from build123d import *

# Parameters (mm, degrees)
F0_W     = 200.66
F0_H     = 200.66
F1_DEPTH = 3.175


# Not quite as in the source:
# - a length typed as a fraction of an inch, garbled in the dataset ("3 / 203.2 mm" for 3/8 in), is restored


with BuildPart() as f1:
    # F0 (on Top) → F1 (new body)
    with BuildSketch(Plane.XY):
        Rectangle(F0_W, F0_H)
        with BuildLine():
            Line((-6.4755703305, -37.973), (-6.4755703305, -38.227))
            ThreePointArc((-6.4755703305, -38.227), (-14.2002143688, -48.9498629888), (-26.715108043, -44.704))
            Line((-26.715108043, -44.704), (-30.0367761716, -44.704))
            Line((-30.0367761716, -44.704), (-44.4783061624, -44.704))
            ThreePointArc((-44.4783061624, -44.704), (-49.0582367841, -42.8069306217), (-50.9553061624, -38.227))
            Line((-50.9553061624, -38.227), (-50.9553061624, -37.973))
            ThreePointArc((-50.9553061624, -37.973), (-49.0582367841, -33.3930693783), (-44.4783061624, -31.496))
            Line((-44.4783061624, -31.496), (-30.0367761716, -31.496))
            Line((-30.0367761716, -31.496), (-26.715108043, -31.496))
            ThreePointArc((-26.715108043, -31.496), (-14.2002143688, -27.2501370112), (-6.4755703305, -37.973))
        make_face(mode=Mode.SUBTRACT)
        with BuildLine():
            Line((82.4244296695, -37.973), (82.4244296695, -38.227))
            ThreePointArc((82.4244296695, -38.227), (74.6997856312, -48.9498629888), (62.184891957, -44.704))
            Line((62.184891957, -44.704), (58.8632238284, -44.704))
            Line((58.8632238284, -44.704), (44.4216938376, -44.704))
            ThreePointArc((44.4216938376, -44.704), (39.8417632159, -42.8069306217), (37.9446938376, -38.227))
            Line((37.9446938376, -38.227), (37.9446938376, -37.973))
            ThreePointArc((37.9446938376, -37.973), (39.8417632159, -33.3930693783), (44.4216938376, -31.496))
            Line((44.4216938376, -31.496), (58.8632238284, -31.496))
            Line((58.8632238284, -31.496), (62.184891957, -31.496))
            ThreePointArc((62.184891957, -31.496), (74.6997856312, -27.2501370112), (82.4244296695, -37.973))
        make_face(mode=Mode.SUBTRACT)
        with BuildLine():
            ThreePointArc((-50.9553061624, 38.227), (-49.0582367841, 42.8069306217), (-44.4783061624, 44.704))
            Line((-44.4783061624, 44.704), (-30.0367761716, 44.704))
            Line((-30.0367761716, 44.704), (-26.715108043, 44.704))
            ThreePointArc((-26.715108043, 44.704), (-14.2002143688, 48.9498629888), (-6.4755703305, 38.227))
            Line((-6.4755703305, 38.227), (-6.4755703305, 37.973))
            ThreePointArc((-6.4755703305, 37.973), (-14.2002143688, 27.2501370112), (-26.715108043, 31.496))
            Line((-26.715108043, 31.496), (-30.0367761716, 31.496))
            Line((-30.0367761716, 31.496), (-44.4783061624, 31.496))
            ThreePointArc((-44.4783061624, 31.496), (-49.0582367841, 33.3930693783), (-50.9553061624, 37.973))
            Line((-50.9553061624, 37.973), (-50.9553061624, 38.227))
        make_face(mode=Mode.SUBTRACT)
        with BuildLine():
            Line((82.4244296695, 38.227), (82.4244296695, 37.973))
            ThreePointArc((82.4244296695, 37.973), (74.6997856312, 27.2501370112), (62.184891957, 31.496))
            Line((62.184891957, 31.496), (58.8632238284, 31.496))
            Line((58.8632238284, 31.496), (44.4216938376, 31.496))
            ThreePointArc((44.4216938376, 31.496), (39.8417632159, 33.3930693783), (37.9446938376, 37.973))
            Line((37.9446938376, 37.973), (37.9446938376, 38.227))
            ThreePointArc((37.9446938376, 38.227), (39.8417632159, 42.8069306217), (44.4216938376, 44.704))
            Line((44.4216938376, 44.704), (58.8632238284, 44.704))
            Line((58.8632238284, 44.704), (62.184891957, 44.704))
            ThreePointArc((62.184891957, 44.704), (74.6997856312, 48.9498629888), (82.4244296695, 38.227))
        make_face(mode=Mode.SUBTRACT)
    extrude(amount=F1_DEPTH)


solid = f1.part
The listing builds one solid part. Answer for the finished solid, in the listing's coordinates (mm). A direction names the side the tool comes from. Coordinates: 2 decimals unless noted, no trailing zeros. Order: outer loops, then holes, each group sorted by start corner. A loop starts at its lowest first (then second) coordinate and runs counter-clockwise, first axis right, second up. Notation, with made-up numbers: (76.25, 31) -> (117.25, 31) arc R28 ccw to (117.25, 67) -> close; hole circle Ø6 at (17.5, -12). An arc over 180 degrees is marked (long way). Answer in a Markdown table with one row per item. Add a question column.
Item 1: Find the intervals of material crossed by L1, parallel to Y at x = -18.5, z = 2.3; L2, parallel to Y at x = 43, z = 0.2, in increasing order. Write a range as from..to.
Item 2: Which of the six approach directions +Z, -Z, +X, -X, +Y, -Y give full straight-line access (tool end or side, diameter ignored) to faces 3 (the face through (74.888, 27.312, 1.565)), 4 (the face through (-1, 1, 0))?
Item 3: Find section B-B (z = 0.5). State how many separate pieces and enclosed holes the cut face has, then the cut area to 3 significant figures.
Item 4: Determine the mould class of faces 1 (the face through (39.792, -33.444, 1.565)), 2 (the face through (-1, 1, 3.175)) for opening direction Y: +Y half, -Y half, draft (parallel to the pull), parting line (faces both ways), or undercut.
Item 5: Find section A-A (x = 58.5). Write down the section's boundary in (y, z) (3 decimals), then the cut area to 3 significant figures.
Result set:
| question | item | result |
|---|---|---|
| 1 | L1 | y = -100.33..-49.44, -26.76..26.76, 49.44..100.33 |
| 1 | L2 | y = -100.33..-44.55, -31.65..31.65, 44.55..100.33 |
| 2 | face 3 | +Z, -Z |
| 2 | face 4 | -Z, +X, -X, +Y, -Y |
| 3 | separate pieces | 1 |
| 3 | enclosed holes | 4 |
| 3 | area | 37,500 mm² |
| 4 | face 1 | undercut |
| 4 | face 2 | draft |
| 5 | outline | (-100.33, 0) -> (-44.704, 0) -> (-44.704, 3.175) -> (-100.33, 3.175) -> close; (-31.496, 0) -> (31.496, 0) -> (31.496, 3.175) -> (-31.496, 3.175) -> close; (44.704, 0) -> (100.33, 0) -> (100.33, 3.175) -> (44.704, 3.175) -> close |
| 5 | area | 553 mm² |
